Read the model definition and answer for the solid it produces. Units are mm, in the model's axes. A direction names the side the tool comes from. Give positions to 0.01 mm unless a question says otherwise; leave off trailing zeros. Loops run counter-clockwise (first coordinate to the right, second up) from the corner with the lowest first, then second, coordinate; pieces in that order, holes last. Notation, with made-up numbers: (50, 23) - (99, 23) arc R22 ccw to (99, 47) - close; hole circle Ø5 at (25, 13.25). An arc over 180 degrees is marked (long way). Put each result on its own line as item: value. Start each with the question number.
1. Consider L1, parallel to Z at x = 0, y = 3.1; L2, parallel to Y at x = 1.5, z = -11; L3, parallel to Z at x = 0, y = 1.9. Determine where each line is inside the solid, lowest interval first. Write a range as from..to.
2. For faces 1 (the flat face through (0.7, 0, -2.3)), 2 (the cylindrical face through (0, 3, -16)), 3 (the flat face through (-2.8, 3, 8)), 4 (the flat face through (0, 2.7, 0)), 5 (the flat face through (2.8, 3, 8)), determine the directions among +Z, -Z, +X, -X, +Y, -Y from which every point of the face is accessible in a straight line to the end or side of a thin tool.
3. A cutting plane is placed at C-C, the plane z = 12.5. Determine the outline of the cut face in (x, y).
4. For a pull along X with two mould halves and no side action, classify faces 6 (the cylindrical face through (-0.29, 1.33, 2.23)), 7 (the flat face through (2.8, 3, -8)), 8 (the flat face through (-2.8, 3, -8)) as released by +X, released by -X, zero draft, split by the parting line, or undercut.
5. Given pin 1 Ø3 at (x, z) = (0.5, -10) entering from -Y; pin 2 Ø1.2 at (y, z) = (3.5, -6) entering from -X; pin 3 Ø0.8 at (y, z) = (3, -6.5) entering from +X, each flat-ended and moving along its own axis, determine where each tip first touches the part or whether it passes through.
6. A cutting plane is placed at A-A, the plane x = 0. Determine the outline of the cut face in (y, z), plus the area to 4 significant figures.
7. A cutting plane is placed at D-D, the plane z = 1. Determine the outline of the cut face in (x, y), plus the area to 3 significant figures.
8. A cutting plane is placed at B-B, the plane y = 3.55. Determine the outline of the cut face in (x, z), plus the area to 3 significant figures.
```python
from build123d import *

# Parameters (mm, degrees)
F0_R     = 3.5
F1_DEPTH = 4.2
F3_DEPTH = 1.5
F4_R     = 0.5
F5_DEPTH = 25
F6_R     = 2.25
F7_DEPTH = 2.7


with BuildPart() as f1:
    # F0 (on Front) → F1 (new body)
    with BuildSketch(Plane.XZ):
        Circle(F0_R)
    extrude(amount=-F1_DEPTH)

    # F2 (on face) → F3 (join)
    with BuildSketch(Plane(origin=(0, 4.2, 0), x_dir=(-1, 0, 0), z_dir=(0, 1, 0))):
        with BuildLine():
            ThreePointArc((2.8, 13.2), (0, 16), (-2.8, 13.2))
            Line((-2.8, 13.2), (-2.8, -13.2))
            ThreePointArc((-2.8, -13.2), (0, -16), (2.8, -13.2))
            Line((2.8, -13.2), (2.8, 13.2))
        make_face()
    extrude(amount=-F3_DEPTH)

    # F4 (on face) → F5 (cut)
    with BuildSketch(Plane.XZ.offset(-2.7)):
        with Locations((0, 12.5)):
            Circle(F4_R)
        with Locations((0, -12.5)):
            Circle(F4_R)
    extrude(amount=-F5_DEPTH, mode=Mode.SUBTRACT)

    # F6 (on face) → F7 (cut)
    with BuildSketch(Plane.XZ):
        Circle(F6_R)
    extrude(amount=-F7_DEPTH, mode=Mode.SUBTRACT)


solid = f1.part
```
Return value:
1. L1: z = -16..-13, -12..12, 13..16
1. L2: y = 2.7..4.2
1. L3: z = -3.5..-2.25, 2.25..3.5
2. face 1: +Z, -Z, +X, -X, -Y
2. face 2: -Z, +Y, -Y
2. face 3: +Z, -X, +Y, -Y
2. face 4: -Y
2. face 5: +Z, +X, +Y, -Y
3. outline: (-2.8, 2.7) - (-0.5, 2.7) - (-0.5, 4.2) - (-2.8, 4.2) - close; (0.5, 2.7) - (2.8, 2.7) - (2.8, 4.2) - (0.5, 4.2) - close
4. face 6: undercut
4. face 7: released by +X
4. face 8: released by -X
5. pin 1: stops at y = 2.7
5. pin 2: stops at x = -2.8
5. pin 3: stops at x = 2.8
6. outline: (0, -3.5) - (2.7, -3.5) - (2.7, -12) - (4.2, -12) - (4.2, 12) - (2.7, 12) - (2.7, 3.5) - (0, 3.5) - (0, 2.25) - (2.7, 2.25) - (2.7, -2.25) - (0, -2.25) - close; (2.7, -16) - (4.2, -16) - (4.2, -13) - (2.7, -13) - close; (2.7, 13) - (4.2, 13) - (4.2, 16) - (2.7, 16) - close
6. area: 51.75 mm2
7. outline: (-3.35, 0) - (-2.02, 0) - (-2.02, 2.7) - (2.02, 2.7) - (2.02, 0) - (3.35, 0) - (3.35, 4.2) - (-3.35, 4.2) - close
7. area: 17.3 mm2
8. outline: (-2.8, -13.2) arc R2.8 ccw to (2.8, -13.2) - (2.8, -2.1) arc R3.5 ccw to (2.8, 2.1) - (2.8, 13.2) arc R2.8 ccw to (-2.8, 13.2) - (-2.8, 2.1) arc R3.5 ccw to (-2.8, -2.1) - close; hole circle Ø1 at (0, -12.5); hole circle Ø1 at (0, 12.5)
8. area: 175 mm2
